Part model, mm, in its own coordinate system. Face numbers are marked on the shaded views. A direction names the side the tool comes from. Coordinates: 2 decimals unless noted, no trailing zeros. Order: outer loops, then holes, each group sorted by start corner. A loop starts at its lowest first (then second) coordinate and runs counter-clockwise, first axis right, second up.
Autodesk Inventor part; units mm, degrees
ref_plane "Work Plane1" through (0, 0, -15) normal (0, 0, 1) x (1, 0, 0)
ref_plane "YZ Plane" through (0, 0, 0) normal (1, 0, 0) x (0, 1, 0)
ref_plane "XZ Plane" through (0, 0, 0) normal (0, 1, 0) x (-1, 0, 0)
sketch "Sketch1" plane through (0, 0, 0) normal (0, 0, 1) x (1, 0, 0)
  line L0 (0, 0) -> (25, 0)
  line L1 (25, 0) -> (25, 40)
  line L2 (25, 40) -> (0, 40)
  line L3 (0, 40) -> (0, 0)
  dimension "d1" = 25
  dimension "d2" = 40
  dimension "d3" = 25
extrude "Extrusion1" add sketch "Sketch1" against normal blind 30
sketch "Sketch2" plane through (25, 0, 0) normal (1, 0, 0) x (0, 0, -1)
  line L0 (0, 0) -> (30, 0)
  circle A0 centre (15, 6.56) radius 2.46
extrude "Extrusion2" cut sketch "Sketch2" against normal blind 30
sketch "Sketch3" plane through (0, 0, 0) normal (-1, 0, 0) x (0, 0, 1)
  line L0 (0, 0) -> (-30, 0)
  line L1 (-25.05, 0) -> (-4.95, 0)
  line L2 (-4.95, 0) -> (-4.95, 33.12)
  line L3 (-4.95, 33.12) -> (-25.05, 33.12)
  line L4 (-25.05, 33.12) -> (-25.05, 0)
  dimension "d11" = 20.1
extrude "Extrusion3" cut sketch "Sketch3" against normal blind 20
sketch "Sketch4" plane through (0, 0, 0) normal (0, -1, 0) x (1, 0, 0)
  line L0 (20, -4.95) -> (20, -25.05)
  line L1 (20, -15) -> (25, -15)
  line L2 (25, 0) -> (25, -30)
  line L3 (20, -8.025) -> (25, -8.025)
  line L4 (25, -8.025) -> (25, -21.975)
  line L5 (25, -21.975) -> (20, -21.975)
  line L6 (20, -21.975) -> (20, -8.025)
  line L7 (20, -8.025) -> (25, -21.975) construction
  line L8 (25, -8.025) -> (20, -21.975) construction
  line L9 (25, -12.54) -> (25, -17.46)
  point P0 (0, 0)
  point P1 (22.5, -15)
  dimension "d14" = 13.95
extrude "Extrusion4" add sketch "Sketch4" along normal blind 15
sketch "Sketch5" plane through (20, 0, 0) normal (-1, 0, 0) x (0, 0, 1)
  circle A0 centre (-15, 6.56) radius 2.46
  circle A1 centre (-15, 6.56) radius 4.7025
  circle A2 centre (-15, 6.56) radius 2.46
  circle A3 centre (-15, 6.56) radius 2.46
  point P0 (0, 0)
  dimension "d17" = 9.405
extrude "Extrusion5" cut sketch "Sketch5" against normal blind 2.1
sketch "Sketch6" plane through (25, 0, 0) normal (1, 0, 0) x (0, 0, -1)
  circle A0 centre (15, 6.56) radius 4.7025
  line L0 (15, 6.56) -> (15, 23.56)
  circle A1 centre (15, 23.56) radius 2.46
  point P0 (0, 0)
  dimension "d20" = 17
  dimension "d21" = 4.92
extrude "Extrusion6" cut sketch "Sketch6" against normal blind 10 contours A1
sketch "Sketch7" plane through (20, 0, 0) normal (-1, 0, 0) x (0, 0, 1)
  circle A0 centre (-15, 23.56) radius 2.46
  circle A1 centre (-15, 23.56) radius 4.7025
  point P0 (0, 0)
  dimension "d24" = 9.405
extrude "Extrusion7" cut sketch "Sketch7" against normal blind 2.1
sketch "Sketch9" plane through (25, 0, 0) normal (1, 0, 0) x (0, 0, -1)
  circle A0 centre (15, 6.56) radius 2.46
  circle A1 centre (15, 6.56) radius 2.46
  circle A2 centre (15, 23.56) radius 2.46
  circle A3 centre (15, 23.56) radius 2.46
  line L0 (30, 40) -> (30, 0)
  line L1 (30, 0) -> (30, 40)
  line L2 (30, 40) -> (0, 40)
  line L3 (0, 40) -> (0, 0)
  line L4 (0, 0) -> (8.025, 0)
  line L5 (21.975, 0) -> (21.975, -15)
  line L6 (21.975, -15) -> (8.025, -15)
  line L7 (8.025, -15) -> (8.025, 0)
  line L8 (0, 0) -> (8.025, 0)
  line L9 (21.975, 0) -> (30, 0)
extrude "Extrusion8" add sketch "Sketch9" along normal blind 5
sketch "Sketch10" plane through (0, 40, 0) normal (0, 1, 0) x (1, 0, 0)
  line L0 (0, 30) -> (30, 30)
  line L1 (30, 0) -> (0, 0)
  line L2 (0, 30) -> (30, 30)
  line L3 (30, 30) -> (30, 0)
  line L4 (30, 0) -> (0, 0)
  line L5 (0, 0) -> (0, 30)
extrude "Extrusion9" add sketch "Sketch10" along normal blind 30
sketch "Sketch12" plane through (30, 0, 0) normal (1, 0, 0) x (0, 0, -1)
  circle A0 centre (15, 6.56) radius 2.46
  line L0 (15, 6.56) -> (15, 15.06)
  circle A1 centre (15, 15.06) radius 2.525
  point P0 (0, 0)
  dimension "d31" = 8.5
  dimension "d33" = 5.05
extrude "Extrusion10" cut sketch "Sketch12" against normal blind 30 contours A1
sketch "Sketch14" plane through (0, 0, 0) normal (0, 0, 1) x (1, 0, 0)
  line L0 (30, 70) -> (0, 70)
  line L1 (0, 70) -> (0, 85)
  line L2 (-15, 100) -> (-23, 100)
  line L3 (30, 0) -> (30, 70)
  line L4 (30, 122.5) -> (30, 70)
  arc A0 (0, 85) -> (-15, 100) centre (-15, 85) ccw
  line L5 (30, 105) -> (30, 100)
  line L6 (-23, 145) -> (15, 145)
  line L7 (-18, 142.5) -> (-23, 145)
  line L8 (-18, 102.5) -> (-23, 100)
  line L9 (-18, 102.5) -> (-13, 122.5)
  line L10 (-13, 122.5) -> (-18, 142.5)
  line L11 (30, 122.5) -> (15, 145)
  point P0 (0, 0)
  point P1 (0, 100)
  dimension "d47" = 30
  dimension "d54" = 15
extrude "Extrusion12" add sketch "Sketch14" against normal blind 30
sketch "Sketch15" plane through (0, 0, -25.05) normal (-1, 0, 0) x (0, 0, 1)
  line L0 (0, 33.12) -> (20.1, 33.12)
  line L1 (20.1, 33.12) -> (20.1, 0)
  line L2 (0, 33.12) -> (20.1, 33.12)
  line L3 (20.1, 33.12) -> (20.1, 31.1)
  line L4 (20.1, 31.1) -> (0, 31.1)
  line L5 (0, 31.1) -> (0, 33.12)
  point P0 (25.05, 0)
  dimension "d57" = 2.02
extrude "Extrusion13" add sketch "Sketch15" against normal blind 20
sketch "Sketch24" plane through (0, 0, 0) normal (0, 0, 1) x (1, 0, 0)
  line L0 (-15, 100) -> (-23, 100)
  line L1 (-15, 100) -> (-23, 100)
  line L2 (-23, 100) -> (-18, 102.5)
  line L3 (-23, 100) -> (-18, 102.5)
  line L4 (-18, 102.5) -> (-13, 122.5)
  line L5 (-18, 102.5) -> (-13, 122.5)
  line L6 (-13, 122.5) -> (-18, 142.5)
  line L7 (-13, 122.5) -> (-18, 142.5)
  line L8 (-18, 142.5) -> (-23, 145)
  line L9 (-18, 142.5) -> (-23, 145)
  line L10 (-23, 145) -> (15, 145)
  line L11 (-23, 145) -> (15, 145)
  line L12 (15, 145) -> (30, 122.5)
  line L13 (15, 145) -> (30, 122.5)
  line L14 (30, 122.5) -> (30, 77.5)
  line L15 (30, 0) -> (30, 122.5)
  line L16 (30, 77.5) -> (0, 77.5)
  line L17 (0, 0) -> (0, 85)
  line L18 (0, 77.5) -> (0, 85)
  arc A0 (0, 85) -> (-15, 100) centre (-15, 85) ccw
  arc A1 (0, 85) -> (-15, 100) centre (-15, 85) ccw
  dimension "d86" = 45
extrude "Extrusion14" add sketch "Sketch24" along normal blind 15
ref_plane "Work Plane1" through (0, 0, -15) normal (0, 0, 1) x (1, 0, 0)
mirror "Mirror1" about plane through (0, 0, -15) normal (0, 0, 1) of "Extrusion14"
properties part number "rec_a_40mm_x_60mm"
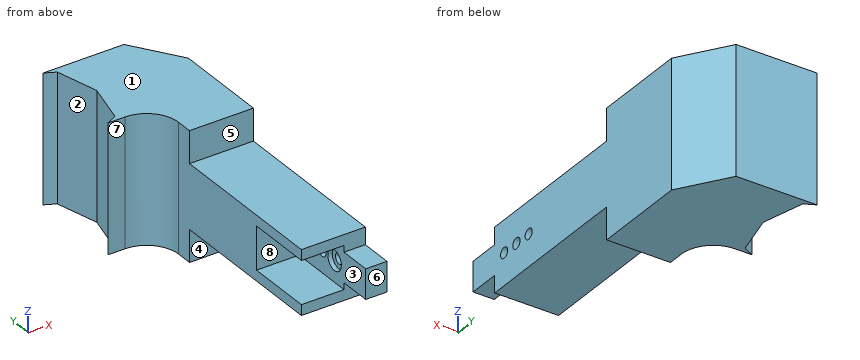
Q1. Cut at C-C on z = -15. Count the separate pieces of the cut face and the enclosed holes in it, and give its area (3 significant figures).
Results list:
separate pieces: 4
enclosed holes: 0
area: 4,310 mm2
Q2. Which spindle directions (+Z, -Z, +X, -X, +Y, -Y) get a long thin tool onto all of the face, cutting with end or side? Do the marked faces 4, 5, 6, 7 and 8. Say none if no direction does.
Results list:
face 4: -Z, +X, -X, -Y
face 5: +Z, +X, -X, -Y
face 6: +Z, -Z, +X, -X, -Y
face 7: +Z, -Z, -X, -Y
face 8: -X, -Y
Q3. Cut at A-A on y = 15.06. Write the cut outline in (x, z) (3 decimals), and give its area (4 significant figures).
Results list:
outline: (0, -30) - (30, -30) - (30, -17.525) - (20, -17.525) - (20, -25.05) - (0, -25.05) - close; (0, -4.95) - (20, -4.95) - (20, -12.475) - (30, -12.475) - (30, 0) - (0, 0) - close
area: 447.5 mm2
Q4. Pin check, flat tips, straight feed: pin 1 Ø15 at (x, y) = (10.5, 55) entering from +Z; pin 2 Ø11 at (x, y) = (26, -8) entering from -Z (3 decimals); pin 3 Ø4.5 at (y, z) = (8, -13.5) entering from -X. Stop position of each tip, or through.
Results list:
pin 1: stops at z = 0
pin 2: stops at z = -21.975
pin 3: stops at x = 22.1
Q5. Wall check: line 1 along Z through (x, y) = (25.75, 15.06) (3 decimals); line 2 along Y through (x, z) = (21, -15) (1 decimal); line 3 along Y through (x, z) = (24, -15) (3 decimals). Give the ranges that are in metal, low to high.
Results list:
line 1: z = -30 to -17.525, -12.475 to 0
line 2: y = -15 to 1.9, 11.3 to 12.5, 17.6 to 18.9, 28.3 to 136
line 3: y = -15 to 4.1, 9.02 to 12.535, 17.585 to 21.1, 26.02 to 131.5
Q6. Cut at D-D on z = -39.5. Write the cut outline in (x, y).
Results list:
outline: (-23, 100) - (-15, 100) arc R15 cw to (0, 85) - (0, 77.5) - (30, 77.5) - (30, 122.5) - (15, 145) - (-23, 145) - (-18, 142.5) - (-13, 122.5) - (-18, 102.5) - close
Q7. Cut at B-B on x = 2. Write the cut outline in (y, z).
Results list:
outline: (0, -30) - (77.5, -30) - (77.5, -45) - (145, -45) - (145, 15) - (77.5, 15) - (77.5, 0) - (0, 0) - (0, -4.95) - (31.1, -4.95) - (31.1, -25.05) - (0, -25.05) - close
Q8. Mould opens along Z. For the marked faces 1, 2 and 3 say: pulls with the +Z half, pulls with the -Z half, needs draft (parallel to the pull), parting line crosses it, or undercut.
Results list:
face 1: pulls with the +Z half
face 2: needs draft
face 3: undercut
